For this review, take the finished solid that the model builds, in its own axes (mm). A direction names the side the tool comes from. Round coordinates to 2 decimals unless told otherwise and drop trailing zeros. Order: outer loops, then holes, each group sorted by start corner. A loop starts at its lowest first (then second) coordinate and runs counter-clockwise, first axis right, second up. Notation, with made-up numbers: M 38,-10 L 61,-10 A12 cw 61,10 Z; hole C 45,-12.5 d2. An arc over 180 degrees is marked long. Use a Markdown table: item, result.
from build123d import *

# Parameters (mm, degrees)
F0_W      = 152.4
F0_H      = 165.1
F1_DEPTH  = 50.8
F3_DEPTH  = 101.6
F5_DEPTH  = 165.101
F7_DEPTH  = 25.4
F8_W      = 5.535897017
F8_H      = 67.31
F9_DEPTH  = 48.222235943
F11_DEPTH = 25.4
F13_DEPTH = 25.4
F14_W     = 60.9961288601
F14_H     = 11.3769355246
F15_DEPTH = 50.8


with BuildPart() as f1:
    # F0 (on Top) → F1 (new body)
    with BuildSketch(Plane.XY):
        with Locations((-76.2, 82.55)):
            Rectangle(F0_W, F0_H)
    extrude(amount=F1_DEPTH)

    # F2 (on face) → F3 (cut)
    with BuildSketch(Plane.YZ):
        Polygon((0, 0), (65.532, 0), (38.608, 46.633735943), (41.357630657, 48.221235943), (67.3650871047, 3.175), (165.1, 3.175), (165.1, 50.8), (0, 50.8), align=None)
    extrude(amount=-F3_DEPTH, mode=Mode.SUBTRACT)

    # F4 (on face) → F5 (cut, through all)
    with BuildSketch(Plane.XZ):
        Polygon((-127.552369343, 48.221235943), (-101.6, 3.2704136641), (-101.6, 50.8), (-152.4, 50.8), (-152.4, 0), (-103.378, 0), (-130.302, 46.633735943), align=None)
    extrude(amount=-F5_DEPTH, mode=Mode.SUBTRACT)

    # F6 (on face) → F7 (cut)
    with BuildSketch(Plane(origin=(-74.783869343, 0, -43.1764870962), x_dir=(0, 1, 0), z_dir=(0.8660254038, 0, 0.5))):
        with BuildLine():
            Line((165.1, 105.537), (146.05, 105.537))
            ThreePointArc((146.05, 105.537), (159.5203841816, 99.9573841816), (165.1, 86.487))
            Line((165.1, 86.487), (165.1, 105.537))
        make_face()
        Polygon((67.31, 105.537), (0, 105.537), (0, 53.632261314), (63.6438257906, 53.632261314), (67.31, 53.632261314), align=None)
    extrude(amount=-F7_DEPTH, mode=Mode.SUBTRACT)

    # F8 (on face) → F9 (cut, through all)
    with BuildSketch(Plane(origin=(0, 0, 0), x_dir=(1, 0, 0), z_dir=(0, 0, -1))):
        with Locations((-106.1459485085, -33.655)):
            Rectangle(F8_W, F8_H)
        Polygon((-101.6, -65.532), (-101.6, 0), (-103.378, 0), (-103.378, -67.31), (-101.6, -67.31), align=None)
    extrude(amount=-F9_DEPTH, mode=Mode.SUBTRACT)

    # F10 (on face) → F11 (cut)
    with BuildSketch(Plane(origin=(0, 51.898630657, 29.9636883804), x_dir=(-1, 0, 0), z_dir=(0, 0.8660254038, 0.5))):
        with BuildLine():
            ThreePointArc((50.8, 2.032), (56.3796158184, 15.5023841816), (69.85, 21.082))
            Line((69.85, 21.082), (0, 21.082))
            Line((0, 21.082), (0, -30.9329128953))
            Line((0, -30.9329128953), (50.8, -30.9329128953))
            Line((50.8, -30.9329128953), (50.8, 2.032))
        make_face()
    extrude(amount=-F11_DEPTH, mode=Mode.SUBTRACT)

    # F12 (on face) → F13 (cut)
    with BuildSketch(Plane.XY.offset(3.175)):
        with BuildLine():
            Line((0, 67.3650871047), (0, 86.4150871047))
            ThreePointArc((0, 86.4150871047), (-5.5796158184, 72.9447029231), (-19.05, 67.3650871047))
            Line((-19.05, 67.3650871047), (0, 67.3650871047))
        make_face()
    extrude(amount=-F13_DEPTH, mode=Mode.SUBTRACT)

    # F14 (on face) → F15 (cut)
    with BuildSketch(Plane.XY.offset(3.175)):
        with Locations((-20.3019355699, 61.6766193424)):
            Rectangle(F14_W, F14_H)
    extrude(amount=-F15_DEPTH, mode=Mode.SUBTRACT)


solid = f1.part
Q1. Add section A-A (z = 16). Write out the cut boundary in (x, y), then the cut area to 3 significant figures.
Determined:
| item | result |
|---|---|
| outline | M -112.62,67.31 L -108.95,67.31 L -108.95,165.1 L -112.62,165.1 Z; M -101.6,56.29 L -50.8,56.29 L -50.8,59.96 L -101.6,59.96 Z |
| area | 545 mm^2 |
Q2. Add section B-B (x = -88). Write out the cut boundary in (y, z) (3 decimals).
Determined:
| item | result |
|---|---|
| outline | M 38.608,46.634 L 65.532,0 L 165.1,0 L 165.1,3.175 L 67.365,3.175 L 41.358,48.221 Z |
Q3. Machinability: for faces 1 (the flat face through (-114.758, 115.52, 26.06)), 2 (the flat face through (-50, 116, 3.175)), 3 (the flat face through (-35, 67.365, 2)), which of the approach directions +Z, -Z, +X, -X, +Y, -Y give a long, thin tool a straight path to every point of the face, cutting with its end or side? Answer none if there is none.
Determined:
| item | result |
|---|---|
| face 1 | +Z, +X, +Y, -Y |
| face 2 | +Z, +X, +Y |
| face 3 | +Z, -Z, +X, -Y |
Q4. Clearance check with flat-ended pins moving along their axes: pin 1 (5 mm diameter, centred on x = -91, y = 61, fed in from -Z); pin 2 (8 mm diameter, centred on x = -23.5, z = 5, fed in from -Y); pin 3 (3 mm diameter, centred on y = 145.5, z = 36, fed in from -X); pin 4 (8 mm diameter, centred on x = -43, z = 15, fed in from -Y). State where each tip first meets the part, or that it passes through.
Determined:
| item | result |
|---|---|
| pin 1 | stops at z = 3.52 |
| pin 2 | stops at y = 67.37 |
| pin 3 | stops at x = -125.03 |
| pin 4 | passes through |
Q5. Wall thickness on line 1 along Y through (x, z) = (-105.5, 9); line 2 along Z through (x, y) = (-77, 106.5) (3 decimals); line 3 along Y through (x, z) = (-24.5, 2.5): over which ranges is each line inside the solid? List them lowest first. Write a range as [from, to].
Determined:
| item | result |
|---|---|
| line 1 | y = [67.31, 165.1] |
| line 2 | z = [0, 3.175] |
| line 3 | y = [67.37, 165.1] |
Q6. Add section C-C (y = 90.5). Write out the cut boundary in (x, z) (3 decimals).
Determined:
| item | result |
|---|---|
| outline | M -130.302,46.634 L -103.378,0 L 0,0 L 0,3.175 L -101.6,3.175 L -101.6,3.27 L -127.552,48.221 Z |
Q7. Add section D-D (y = 75). Write out the cut boundary in (x, z) (3 decimals).
Determined:
| item | result |
|---|---|
| outline | M -130.302,46.634 L -103.378,0 L -3.799,0 L -3.799,3.175 L -101.6,3.175 L -101.6,3.27 L -127.552,48.221 Z |
